```python
from build123d import *

# Parameters (mm, degrees)
SKETCH3_R                   = 4.064
CUT_EXTRUDE1_DEPTH          = 21.32
F_1_4_20_TAPPED_HOLE1_D     = 5.1054
F_1_4_20_TAPPED_HOLE1_DEPTH = 10.16
F_1_4_20_TAPPED_HOLE1_TIP   = 1.533816902
CIRPATTERN1_COUNT           = 3


with BuildPart() as part:
    # Sketch1 → Revolve1 (revolve)
    with BuildSketch(Plane(origin=(0, 0, 0), x_dir=(0, 0, -1), z_dir=(1, 0, 0))):
        Polygon((0, 12.7), (-13.97, 12.7), (-13.97, 25.4), (-20.32, 25.4), (-20.32, 0), (0, 0), align=None)
    revolve(axis=Axis((0, 0, 20.32), (0, 0, -1)))

    # Sketch3 → Cut-Extrude1 (cut, through all)
    with BuildSketch(Plane(origin=(0, 0, 0), x_dir=(-1, 0, 0), z_dir=(0, 0, -1))):
        Circle(SKETCH3_R)
    extrude(amount=-CUT_EXTRUDE1_DEPTH, mode=Mode.SUBTRACT)

    # 1/4-20 Tapped Hole1
    with Locations(Plane(origin=(0, 12.7, 7.62), x_dir=(1, 0, 0), z_dir=(0, 1, 0))):
        with Locations((0, 0)):
            Hole(F_1_4_20_TAPPED_HOLE1_D / 2, depth=F_1_4_20_TAPPED_HOLE1_DEPTH)
            with Locations((0, 0, -(F_1_4_20_TAPPED_HOLE1_DEPTH + F_1_4_20_TAPPED_HOLE1_TIP / 2))):  # 118° drill point
                Cone(0, F_1_4_20_TAPPED_HOLE1_D / 2, F_1_4_20_TAPPED_HOLE1_TIP, mode=Mode.SUBTRACT)

    # Sketch7 → 1/4 (0.25) Diameter Hole1 (revolve, cut)
    with BuildSketch(Plane(origin=(0, 19.05, 13.97), x_dir=(0, 1, 0), z_dir=(1, 0, 0))):
        Polygon((0, 0), (0, 20.957732465), (3.175, 19.05), (3.175, 0), align=None)
    f_1_4_0_25_diameter_hole1 = revolve(axis=Axis((0, 19.05, 7.62), (0, 0, 1)), mode=Mode.SUBTRACT)

    # CirPattern1: 1/4 (0.25) Diameter Hole1 ×3 about axis
    cirpattern1_axis = Axis((0, 0, 0), (0, 0, 1))
    for i in range(1, CIRPATTERN1_COUNT):
        add(f_1_4_0_25_diameter_hole1.rotate(cirpattern1_axis, i * 360 / CIRPATTERN1_COUNT), mode=Mode.SUBTRACT)


solid = part.part
```
Input: part model. Units: mm. Frame: model coordinates. A direction names the side the tool comes from. Give positions to 0.01 mm unless a question says otherwise; leave off trailing zeros. Loops run counter-clockwise (first coordinate to the right, second up) from the corner with the lowest first, then second, coordinate; pieces in that order, holes last.
1) Mould query, pull axis Y, two halves, no side actions, for faces 4 (the flat face through (0, 5, 20.32)), 5 (the cylindrical face through (-12.4, -2.75, 7.08)), 6 (the cylindrical face through (-0.14, 15.88, 17.1)). Classes: released by +Y, released by -Y, zero draft, split by the parting line, or undercut.
A:
face 4: zero draft
face 5: split by the parting line
face 6: undercut
2) Contact query for flat-ended pins moving along their axis: pin 1 (3 mm diameter, centred on x = 0, z = 7.62, fed in from +Y); pin 2 (6 mm diameter, centred on y = 13, z = 14.5, fed in from -X); pin 3 (3 mm diameter, centred on y = -2.5, z = 8, fed in from -X). Output: stop coordinate, or through.
A:
pin 1: stops at y = -3.78
pin 2: stops at x = -23.35
pin 3: stops at x = -12.66
3) Section query B-B on y = 0. Return the cut outline in (x, z), and give its area (3 significant figures).
A:
outline: (-25.4, 13.97) - (-12.7, 13.97) - (-12.7, 0) - (-4.06, 0) - (-4.06, 20.32) - (-25.4, 20.32) - close; (4.06, 0) - (12.7, 0) - (12.7, 13.97) - (25.4, 13.97) - (25.4, 20.32) - (4.06, 20.32) - close
area: 512 mm2
4) Section query A-A on x = 0. Return the cut outline in (y, z) (3 decimals), and give its area (3 significant figures).
A:
outline: (-25.4, 13.97) - (-12.7, 13.97) - (-12.7, 0) - (-4.064, 0) - (-4.064, 20.32) - (-25.4, 20.32) - close; (4.064, 0) - (12.7, 0) - (12.7, 5.067) - (4.064, 5.067) - close; (4.064, 10.173) - (12.7, 10.173) - (12.7, 13.97) - (15.875, 13.97) - (15.875, 20.32) - (4.064, 20.32) - close; (22.225, 13.97) - (25.4, 13.97) - (25.4, 20.32) - (22.225, 20.32) - close
area: 428 mm2
5) Section query D-D on z = 17.75. Count the separate pieces of the cut face and the enclosed holes in it, and give its area (3 significant figures).
A:
separate pieces: 1
enclosed holes: 4
area: 1,880 mm2
6) Line query: L1, parallel to Z at x = 0, y = 6.75; L2, parallel to Z at x = 8.5, y = -16; L3, parallel to X at y = 19.05, z = 19.25 (3 decimals). Output: solid intervals per line, ascending.
A:
L1: z = 0 to 5.07, 10.17 to 20.32
L2: z = 13.97 to 20.32
L3: x = -16.801 to -3.175, 3.175 to 16.801
7) Reachability of faces 1 (the flat face through (3, 3, 0)), 2 (the cylindrical face through (2.55, 7.86, 7.51)), 3 (the flat face through (-5, 12, 13.97)) from +Z, -Z, +X, -X, +Y, -Y: full face, straight path, thin tool, end or side. Return the list, or none.
A:
face 1: -Z, +X, -X, +Y, -Y
face 2: +Y
face 3: -Z
8) Section query C-C on z = 2. Return the cut outline in (x, y).
A:
outline: circle Ø25.4 at (0, 0); hole circle Ø8.13 at (0, 0)
